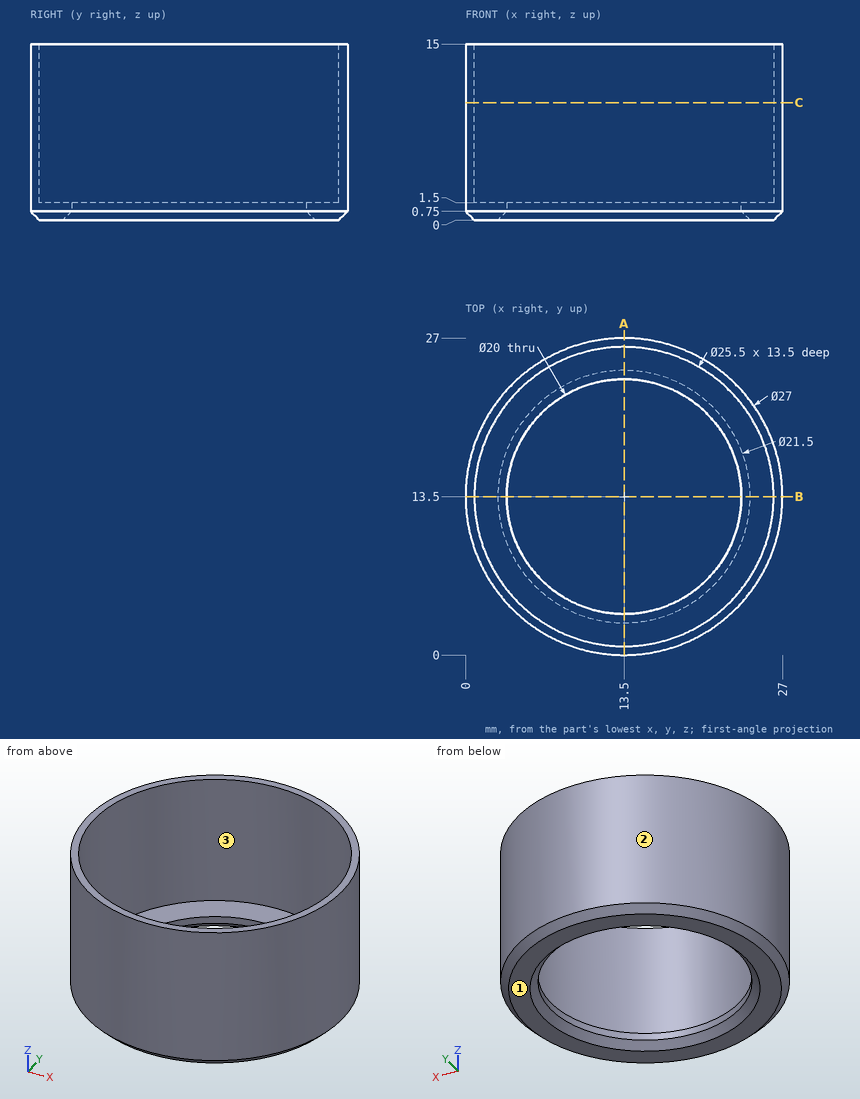
Source: three-view drawing plus pictorial views. Frame: mm from the lowest corner of the part. Round coordinates to 2 decimals unless told otherwise and drop trailing zeros. Write each loop counter-clockwise with the first axis right and the second up, starting at its lowest first coordinate (ties: lowest second). Pieces come first, ordered by that corner, then holes. Notation, with made-up numbers: (-5.5, -20) -> (6.5, -20) arc R23 cw to (6.5, 0) -> close; hole circle Ø10 at (-1, -34.5). An arc over 180 degrees is marked (long way). Return JSON: item names as keys, results as strings.
Q1. Section C-C on z = 10. Return the cut outline in (x, y).
From the geometry:
{"outline": "circle Ø27 at (13.5, 13.5); hole circle Ø25.5 at (13.5, 13.5)"}
Q2. First-contact query: pin 1 Ø1.5 at (x, z) = (19, 6.5) entering from -Y; pin 2 Ø5 at (y, z) = (9.5, 8) entering from +X; pin 3 Ø4 at (y, z) = (24, 12) entering from +X. Flat tips, straight axial feed; report the tip coordinate or a pass-through.
From the geometry:
{"pin 1": "y = 0.86", "pin 2": "x = 26.92", "pin 3": "x = 23.99"}
Q3. Ray query, line 1 (Y direction, x = 13.5, z = 1.05); line 2 (X direction, y = 3.75, z = 3.5); line 3 (Y direction, x = 8, z = 14.5). Return the intervals inside material, ascending.
From the geometry:
{"line 1": "0 to 3.5, 23.5 to 27", "line 2": "4.16 to 5.28, 21.72 to 22.84", "line 3": "1.17 to 2, 25 to 25.83"}
Q4. Mould query, pull axis Y, two halves, no side actions, for the marked faces 1, 2 and 3. Classes: +Y half, -Y half, draft (parallel to the pull), parting line (faces both ways), or undercut.
From the geometry:
{"face 1": "draft", "face 2": "parting line", "face 3": "undercut"}
Q5. Section A-A on x = 13.5. Return the cut outline in (y, z).
From the geometry:
{"outline": "(0, 0.75) -> (0.75, 0) -> (2.75, 0) -> (3.5, 0.75) -> (3.5, 1.5) -> (0.75, 1.5) -> (0.75, 15) -> (0, 15) -> close; (23.5, 0.75) -> (24.25, 0) -> (26.25, 0) -> (27, 0.75) -> (27, 15) -> (26.25, 15) -> (26.25, 1.5) -> (23.5, 1.5) -> close"}
